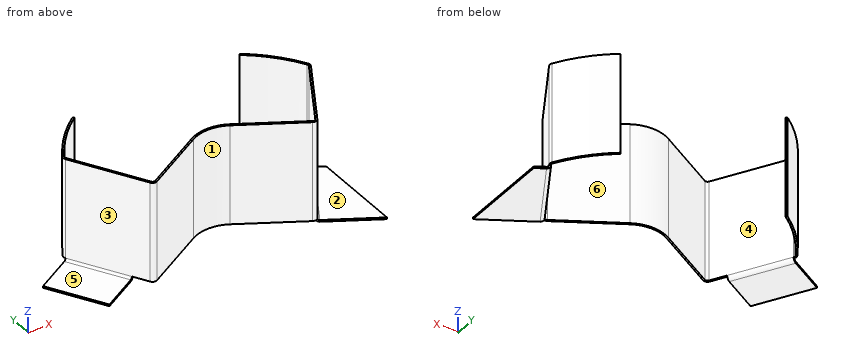
from build123d import *

# Parameters (mm, degrees)
BASE_FLANGE1_DEPTH      = 46.19
BASE_FLANGE1_DEPTH_BACK = 0.8128
EDGE_FLANGE1_DEPTH      = 29
EDGE_FLANGE1_BEND_DEPTH = 37
EDGE_FLANGE1_START      = 0.8128
EDGE_FLANGE1_FLAT_DEPTH = 0.8128


# Sheet-metal steps are written as plain solids
with BuildPart() as part:
    # Sketch1 → Base-Flange1 (new, two sides: drawn at the far end of the back side and taken through both)
    with BuildSketch(Plane.XY.offset(-BASE_FLANGE1_DEPTH_BACK)):
        with BuildLine():
            ThreePointArc((145.409019443, 88.185), (155.762419921, 78.86409034), (163.964489977, 67.603614987))
            ThreePointArc((163.964489977, 67.603614987), (164.234222289, 66.60231267), (163.96627389, 65.600531503))
            Line((163.96627389, 65.600531503), (145.46627389, 33.557591563))
            ThreePointArc((145.46627389, 33.557591563), (144.251861173, 32.625739911), (142.734223083, 32.825540756))
            Line((142.734223083, 32.825540756), (114.675, 49.025540756))
            ThreePointArc((114.675, 49.025540756), (106, 51.35), (97.325, 49.025540756))
            Line((97.325, 49.025540756), (69.265776917, 32.825540756))
            ThreePointArc((69.265776917, 32.825540756), (67.748138827, 32.625739911), (66.53372611, 33.557591563))
            Line((66.53372611, 33.557591563), (48.03372611, 65.600531503))
            ThreePointArc((48.03372611, 65.600531503), (47.76577771, 66.60231267), (48.035510023, 67.603614987))
            ThreePointArc((48.035510023, 67.603614987), (56.237580079, 78.86409034), (66.590980557, 88.185))
            Line((66.590980557, 88.185), (67.069060372, 87.52766939))
            ThreePointArc((67.069060372, 87.52766939), (56.841259359, 78.319833814), (48.738690489, 67.195961859))
            ThreePointArc((48.738690489, 67.195961859), (48.578577388, 66.601588804), (48.737631558, 66.006931503))
            Line((48.737631558, 66.006931503), (67.237631558, 33.963991563))
            ThreePointArc((67.237631558, 33.963991563), (67.958506947, 33.410844422), (68.859376917, 33.529446204))
            Line((68.859376917, 33.529446204), (96.9186, 49.729446204))
            ThreePointArc((96.9186, 49.729446204), (106, 52.1628), (115.0814, 49.729446204))
            Line((115.0814, 49.729446204), (143.140623083, 33.529446204))
            ThreePointArc((143.140623083, 33.529446204), (144.041493053, 33.410844422), (144.762368442, 33.963991563))
            Line((144.762368442, 33.963991563), (163.262368442, 66.006931503))
            ThreePointArc((163.262368442, 66.006931503), (163.421422612, 66.601588804), (163.261309511, 67.195961859))
            ThreePointArc((163.261309511, 67.195961859), (155.158740641, 78.319833814), (144.930939628, 87.52766939))
            Line((144.930939628, 87.52766939), (145.409019443, 88.185))
        make_face()
    extrude(amount=BASE_FLANGE1_DEPTH + BASE_FLANGE1_DEPTH_BACK)

    # Edge-Flange1 section (across the edge) → Edge-Flange1 (add)
    with BuildSketch(Plane(origin=(48.03372611, 65.600531503, -1.8128), x_dir=(0, 0, 1), z_dir=(0.5000000000000168, -0.866025403784429, 0))):
        with BuildLine():
            Line((-0.8128, 1), (-0.8128, 20))
            Line((-0.8128, 20), (0, 20))
            Line((0, 20), (0, 1))
            ThreePointArc((0, 1), (0.292893219, 0.292893219), (1, 0))
            Line((1, 0), (1, -0.8128))
            ThreePointArc((1, -0.8128), (-0.281843173, -0.281843173), (-0.8128, 1))
        make_face()
    extrude(amount=EDGE_FLANGE1_DEPTH)

    # Edge-Flange1 bend section (across the edge) → Edge-Flange1 bend (add)
    with BuildSketch(Plane(origin=(145.46627389, 33.557591563, -1.8128), x_dir=(0, 0, 1), z_dir=(0.4999999999999994, 0.866025403784439, 0))):
        with BuildLine():
            Line((-0.8128, 1), (0, 1))
            ThreePointArc((0, 1), (0.292893219, 0.292893219), (1, 0))
            Line((1, 0), (1, -0.8128))
            ThreePointArc((1, -0.8128), (-0.281843173, -0.281843173), (-0.8128, 1))
        make_face()
    extrude(amount=EDGE_FLANGE1_BEND_DEPTH)

    # Edge-Flange1 profile (on flange) → Edge-Flange1 flat (add)
    with BuildSketch(Plane(origin=(94.568842026, -54.599346401, -1.8128), x_dir=(0.4999999999999994, 0.866025403784439, 0), z_dir=(0, 0, -1)).offset(EDGE_FLANGE1_START)):
        Polygon((101.794863729, 1), (138.794863729, 1), (138.794863729, 6), (101.794863729, 27.36195996), align=None)
    extrude(amount=-EDGE_FLANGE1_FLAT_DEPTH)


solid = part.part
Model file for the job. Use its own axes, mm. Face numbers are marked on the shaded views. A direction names the side the tool comes from. Coordinates: 2 decimals unless noted, no trailing zeros. Write each loop counter-clockwise with the first axis right and the second up, starting at its lowest first coordinate (ties: lowest second). Pieces come first, ordered by that corner, then holes. Notation, with made-up numbers: (7, 52) -> (55, 52) arc R25 cw to (55, 66) -> close; hole circle Ø4 at (27, 41). An arc over 180 degrees is marked (long way). One line per item, written item: value. Start each with the question number.
1) Flat gauge pins, fed straight in: pin 1 Ø1.5 at (x, z) = (140.5, 36) entering from +Y; pin 2 Ø1.5 at (x, z) = (112.5, 27.5) entering from +Y; pin 3 Ø6 at (x, z) = (140, 3) entering from -Y; pin 4 Ø2 at (x, y) = (53, 32.5) entering from +Z. Where does each tip first touch, or does it go through?
2) Slice it at B-B on z = 27.5. Write the cut outline in (x, y) (3 decimals).
3) Probe probe 1 along X at (y, z) = (36, 12); probe 2 along X at (y, z) = (40, 22.5); probe 3 along Y at (x, z) = (50, 12). List the from-to ranges inside material, lowest first.
4) Slice it at C-C on y = 77. Write the cut outline in (x, z).
5) Slice it at A-A on y = 84. Write the cut outline in (x, z).
6) Pull direction X, two halves, no side cores. Call the marked faces 1, 2 and 3: +X half, -X half, draft (parallel to the pull), parting line (faces both ways), or undercut.
7) Slice it at D-D on x = 41. Write the cut outline in (y, z), then the cut area to 3 significant figures.
8) Which spindle directions (+Z, -Z, +X, -X, +Y, -Y) get a long thin tool onto all of the face, cutting with end or side? Do the marked faces 4, 5 and 6. Say none if no direction does.
Answers follow:
1. pin 1: y = 35.49
1. pin 2: y = 51.23
1. pin 3: y = 32.7
1. pin 4: through
2. outline: (48.034, 65.601) -> (66.534, 33.558) arc R2 ccw to (69.266, 32.826) -> (97.325, 49.026) arc R17.35 cw to (114.675, 49.026) -> (142.734, 32.826) arc R2 ccw to (145.466, 33.558) -> (163.966, 65.601) arc R2 ccw to (163.964, 67.604) arc R67.001 ccw to (145.409, 88.185) -> (144.931, 87.528) arc R66.188 cw to (163.261, 67.196) arc R1.187 cw to (163.262, 66.007) -> (144.762, 33.964) arc R1.187 cw to (143.141, 33.529) -> (115.081, 49.729) arc R18.163 ccw to (96.919, 49.729) -> (68.859, 33.529) arc R1.187 cw to (67.238, 33.964) -> (48.738, 66.007) arc R1.187 cw to (48.739, 67.196) arc R66.188 cw to (67.069, 87.528) -> (66.591, 88.185) arc R67.001 ccw to (48.036, 67.604) arc R2 ccw to start
3. probe 1: 65.12 to 66.06, 73.14 to 74.76, 137.24 to 138.86, 145.94 to 146.88
3. probe 2: 62.81 to 63.75, 80.07 to 81.69, 130.31 to 131.93, 148.25 to 149.19
3. probe 3: 62.19 to 63.82, 69.28 to 70.78
4. outline: (54.62, -0.81) -> (55.68, -0.81) -> (55.68, 46.19) -> (54.62, 46.19) -> close; (156.32, -0.81) -> (157.38, -0.81) -> (157.38, 46.19) -> (156.32, 46.19) -> close
5. outline: (61.4, -0.81) -> (62.63, -0.81) -> (62.63, 46.19) -> (61.4, 46.19) -> close; (149.37, -0.81) -> (150.6, -0.81) -> (150.6, 46.19) -> (149.37, 46.19) -> close
6. face 1: undercut
6. face 2: draft
6. face 3: -X half
7. outline: (37.78, -2.63) -> (61.54, -2.63) -> (61.54, -1.81) -> (37.78, -1.81) -> close
7. area: 19.3 mm2
8. face 4: +Z, -Z
8. face 5: +Z, -X, -Y
8. face 6: +Z, -Z, +Y
